```python
from build123d import *

# Parameters (mm, degrees)
SKETCH1_R           = 13.335
SKETCH1_R_2         = 10.4648
BOSS_EXTRUDE1_DEPTH = 177.8
SKETCH1_2_R         = 10.4648
BOSS_EXTRUDE2_DEPTH = 3.175
SKETCH3_R           = 3.175
CUT_EXTRUDE1_DEPTH  = 14.351


with BuildPart() as part:
    # Sketch1 → Boss-Extrude1 (new body)
    with BuildSketch(Plane(origin=(0, 0, 0), x_dir=(1, 0, 0), z_dir=(0, 1, 0))):
        Circle(SKETCH1_R)
        Circle(SKETCH1_R_2, mode=Mode.SUBTRACT)
    extrude(amount=BOSS_EXTRUDE1_DEPTH)

    # Sketch1<2> → Boss-Extrude2 (add)
    with BuildSketch(Plane(origin=(0, 0, 0), x_dir=(1, 0, 0), z_dir=(0, 1, 0))):
        Circle(SKETCH1_2_R)
    extrude(amount=BOSS_EXTRUDE2_DEPTH)

    # Sketch3 → Cut-Extrude1 (cut)
    with BuildSketch(Plane(origin=(13.335, 0, 0), x_dir=(0, 0, -1), z_dir=(1, 0, 0))):
        with Locations((0, 6.35)):
            Circle(SKETCH3_R)
    extrude(amount=-CUT_EXTRUDE1_DEPTH, mode=Mode.SUBTRACT)


solid = part.part
```
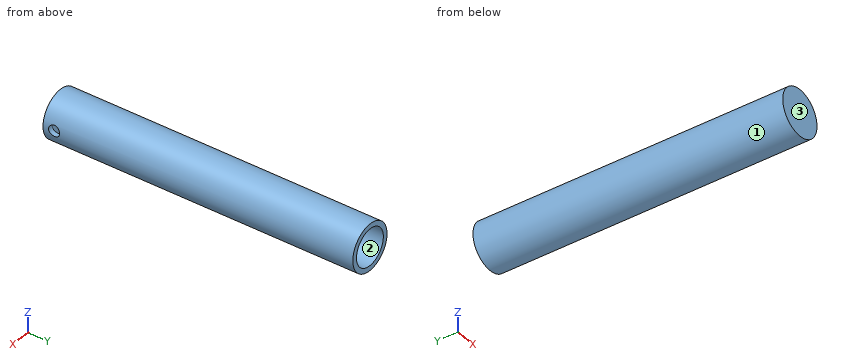
Build history of the part. All positions in model axes, mm. Face numbers are marked on the shaded views. Coordinates: 2 decimals unless noted, no trailing zeros. Write each loop counter-clockwise with the first axis right and the second up, starting at its lowest first coordinate (ties: lowest second). Pieces come first, ordered by that corner, then holes.
1. Band-saw the part on C-C, the plane z = 7. Give the cut face in (x, y) (3 decimals), and give its area (3 significant figures).
Answer block:
outline: (-11.35, 0) - (11.35, 0) - (11.35, 177.8) - (7.779, 177.8) - (7.779, 3.175) - (-7.779, 3.175) - (-7.779, 177.8) - (-11.35, 177.8) - close
area: 1,320 mm2
2. Pull direction Z, two halves, no side cores. Call the marked faces 1, 2 and 3: released by +Z, released by -Z, zero draft, split by the parting line, or undercut.
Answer block:
face 1: split by the parting line
face 2: undercut
face 3: zero draft
3. Band-saw the part on A-A, the plane y = 15. Give the cut face in (x, z) (3 decimals).
Answer block:
outline: circle Ø26.67 at (0, 0); hole circle Ø20.93 at (0, 0)
4. Band-saw the part on B-B, the plane x = -4.75. Give the cut face in (y, z) (3 decimals), and give its area (3 significant figures).
Answer block:
outline: (0, -12.46) - (177.8, -12.46) - (177.8, -9.325) - (3.175, -9.325) - (3.175, 9.325) - (177.8, 9.325) - (177.8, 12.46) - (0, 12.46) - close
area: 1,170 mm2
5. Drill centre lines: probe 1 along X at (y, z) = (39, 0) (3 decimals); probe 2 along Y at (x, z) = (11, 0) (3 decimals). Where is each one in solid material? Low to high.
Answer block:
probe 1: x = -13.335 to -10.465, 10.465 to 13.335
probe 2: y = 0 to 3.175, 9.525 to 177.8
6. Drop flat-ended pins along their axis: pin 1 (5 mm diameter, centred on y = 87, z = 6.5, fed in from +X); pin 2 (10 mm diameter, centred on x = 8, z = 5.5, fed in from -Y); pin 3 (1.5 mm diameter, centred on x = -4.5, y = 66, fed in from -Z); pin 4 (5 mm diameter, centred on x = -0.5, z = -4, fed in from +Y) (3 decimals). Give the stop position or say it passes through.
Answer block:
pin 1: stops at x = 12.72
pin 2: stops at y = 0
pin 3: stops at z = -12.8
pin 4: stops at y = 3.175
